```python
from build123d import *

# Parameters (mm, degrees)
EXTRUDE_1_DEPTH           = 50
FILLET_3_R                = 3
FILLET_4_R                = 3
EXTRUDE_4_DEPTH           = 60
EXTRUDE_5_DEPTH           = 62
CUT_EXTRUDE_7_DEPTH       = 63.635852353
CUT_EXTRUDE_7_DEPTH_BACK  = 4
SKETCH_8_R                = 3
EXTRUDE_6_DEPTH           = 25
CUT_EXTRUDE_10_DEPTH      = 67.695202226
CUT_EXTRUDE_10_DEPTH_BACK = 10


with BuildPart() as part:
    # 草图2 → 凸台-拉伸1 (new body)
    with BuildSketch(Plane(origin=(0, 0, 0), x_dir=(1, 0, 0), z_dir=(0, 1, 0))):
        with BuildLine():
            Line((25, -7.5), (22, -7.5))
            Line((22, -7.5), (22, -12.5))
            Line((22, -12.5), (30, -12.5))
            Line((30, -12.5), (30, 7.407682229))
            ThreePointArc((30, 7.407682229), (26.399187572, 8.899187572), (24.907682229, 12.5))
            Line((24.907682229, 12.5), (-25, 12.5))
            ThreePointArc((-25, 12.5), (-26.464466094, 8.964466094), (-30, 7.5))
            Line((-30, 7.5), (-30, -12.5))
            Line((-30, -12.5), (-22, -12.5))
            Line((-22, -12.5), (-22, -7.5))
            Line((-22, -7.5), (-25, -7.5))
            Line((-25, -7.5), (-25, 2.5))
            Line((-25, 2.5), (25, 2.5))
            Line((25, 2.5), (25, -7.5))
        make_face()
    extrude(amount=EXTRUDE_1_DEPTH)

    # 圆角3
    fillet_3_edges = [part.edges().sort_by_distance(p)[0] for p in [
        (-30, 25, -7.5),
        (-25, 25, -12.5),
    ]]
    fillet(fillet_3_edges, radius=FILLET_3_R)

    # 圆角4
    fillet_4_edges = [part.edges().sort_by_distance(p)[0] for p in [
        (24.907682229, 25, -12.5),
        (30, 25, -7.407682229),
    ]]
    fillet(fillet_4_edges, radius=FILLET_4_R)

    # 草图5 → 凸台-拉伸4 (add)
    with BuildSketch(Plane.ZY.offset(30)):
        Polygon((-2.5, 50), (-20.5, 50), (-2.5, 35), align=None)
    extrude(amount=-EXTRUDE_4_DEPTH)

    # 草图7 → 凸台-拉伸5 (add)
    with BuildSketch(Plane.ZY.offset(31)):
        with BuildLine():
            Line((-2.5, 51), (-2.5, 51.591557712))
            Line((-2.5, 51.591557712), (-2.5, 55))
            Line((-2.5, 55), (-3.5, 55))
            Line((-3.5, 55), (-3.5, 52))
            ThreePointArc((-3.5, 52), (-2.792893219, 51.707106781), (-2.5, 51))
        make_face()
        with BuildLine():
            ThreePointArc((-3.5, 50), (-2.792893219, 50.292893219), (-2.5, 51))
            ThreePointArc((-2.5, 51), (-2.792893219, 51.707106781), (-3.5, 52))
            Line((-3.5, 52), (-3.5, 51))
            Line((-3.5, 51), (-4.5, 51))
            ThreePointArc((-4.5, 51), (-4.207106781, 50.292893219), (-3.5, 50))
        make_face()
        with BuildLine():
            Line((-21.5, 50), (-3.5, 50))
            ThreePointArc((-3.5, 50), (-4.207106781, 50.292893219), (-4.5, 51))
            Line((-4.5, 51), (-21.5, 51))
            Line((-21.5, 51), (-21.5, 50))
        make_face()
    extrude(amount=-EXTRUDE_5_DEPTH)

    # 草图8 → 切除-拉伸7 (cut, two sides: drawn at the far end of the back side and taken through both)
    with BuildSketch(Plane(origin=(0, 50, 0), x_dir=(1, 0, 0), z_dir=(0, 1, 0)).offset(-CUT_EXTRUDE_7_DEPTH_BACK)):
        with Locations(Location((-15, 12.5, 0), (0, 0, 90))):
            Circle(SKETCH_8_R)
        with Locations(Location((15, 12.5, 0), (0, 0, 90))):
            Circle(SKETCH_8_R)
    extrude(amount=CUT_EXTRUDE_7_DEPTH + CUT_EXTRUDE_7_DEPTH_BACK, mode=Mode.SUBTRACT)

    # 草图9 → 凸台-拉伸6 (add)
    with BuildSketch(Plane(origin=(0, 0, 0), x_dir=(1, 0, 0), z_dir=(0, 1, 0))):
        with BuildLine():
            Line((-5, -17.5), (5, -17.5))
            ThreePointArc((5, -17.5), (8.535533906, -16.035533906), (10, -12.5))
            Line((10, -12.5), (10, 2.5))
            Line((10, 2.5), (-10, 2.5))
            Line((-10, 2.5), (-10, -12.5))
            ThreePointArc((-10, -12.5), (-8.535533906, -16.035533906), (-5, -17.5))
        make_face()
    extrude(amount=EXTRUDE_6_DEPTH)

    # 草图9<8> → 切除-拉伸10 (cut, two sides: drawn at the far end of the back side and taken through both)
    with BuildSketch(Plane(origin=(0, 0, 0), x_dir=(1, 0, 0), z_dir=(0, 1, 0)).offset(-CUT_EXTRUDE_10_DEPTH_BACK)):
        with BuildLine():
            ThreePointArc((0, -1.5), (-6, -7.5), (0, -13.5))
            Line((0, -13.5), (0, -7.5))
            Line((0, -7.5), (0, -1.5))
        make_face()
        with BuildLine():
            Line((0, -7.5), (0, -13.5))
            ThreePointArc((0, -13.5), (4.242640687, -11.742640687), (6, -7.5))
            ThreePointArc((6, -7.5), (4.242640687, -3.257359313), (0, -1.5))
            Line((0, -1.5), (0, -7.5))
        make_face()
    extrude(amount=CUT_EXTRUDE_10_DEPTH + CUT_EXTRUDE_10_DEPTH_BACK, mode=Mode.SUBTRACT)


solid = part.part
```
Source: CAD feature listing. Evaluate the final solid. Frame: model axes, mm. A direction names the side the tool comes from. Round coordinates to 2 decimals unless told otherwise and drop trailing zeros. Loops run counter-clockwise (first coordinate to the right, second up) from the corner with the lowest first, then second, coordinate; pieces in that order, holes last.
1. Section query A-A on x = 24. Output: boundary loops of the cut face in (y, z).
2. Contact query for flat-ended pins moving along their axis: pin 1 (3 mm diameter, centred on x = -2.5, z = -11, fed in from +Y); pin 2 (3 mm diameter, centred on x = 4, y = 33.5, fed in from +Z); pin 3 (2.5 mm diameter, centred on x = 24.5, y = 28, fed in from +Z); pin 4 (3 mm diameter, centred on x = 15.5, z = -0.5, fed in from -Y). Output: stop coordinate, or through.
3. Ray query, L1, parallel to X at y = 48.25, z = -12.5; L2, parallel to X at y = 30.5, z = 2; L3, parallel to X at y = 5.5, z = 5. Return the intervals inside material, ascending.
4. Section query B-B on z = 11. Output: boundary loops of the cut face in (x, y), and give its area (3 significant figures).
5. Mould query, pull axis X, two halves, no side actions, for faces 5 (the flat face through (0, 30, -2.5)), 6 (the cylindrical face through (8.5, 12.32, 16.07)), 7 (the flat face through (-0.4, 46.5, -16.3)). Classes: released by +X, released by -X, zero draft, split by the parting line, or undercut.
6. Section query C-C on y = 33. Output: boundary loops of the cut face in (x, z) (3 decimals).
7. Section query D-D on x = 15. Output: boundary loops of the cut face in (y, z).
8. Access query for faces 1 (the flat face through (0, 53, -3.5)), 2 (the flat face through (0, 53, -2.5)), 3 (the cylindrical face through (17.93, 48.46, -11.85)), 4 (the cylindrical face through (29.47, 19.97, -6.69)). Directions: +Z, -Z, +X, -X, +Y, -Y. A direction counts if a zero-diameter tool reaches every point of the face in a straight line with its end or side. Return the directions, or none.
Answers below:
1. outline: (0, -12.09) - (42.99, -12.09) - (50, -20.5) - (50, -21.5) - (51, -21.5) - (51, -3.5) - (55, -3.5) - (55, -2.5) - (51, -2.5) arc R1 ccw to (50, -3.5) - (50, -2.5) - (0, -2.5) - close; (0, 7.5) - (50, 7.5) - (50, 12.5) - (0, 12.5) - close
2. pin 1: stops at y = 51
2. pin 2: stops at z = -2.5
2. pin 3: stops at z = 12.5
2. pin 4: passes through
3. L1: x = -30 to -18, -12 to 12, 18 to 30
3. L2: x = -30 to -25, 25 to 30
3. L3: x = -30 to -25, -10 to -5.45, 5.45 to 10, 25 to 30
4. outline: (-30, 0) - (-22, 0) - (-22, 50) - (-30, 50) - close; (-10, 0) - (-4.87, 0) - (-4.87, 25) - (-10, 25) - close; (4.87, 0) - (10, 0) - (10, 25) - (4.87, 25) - close; (22, 0) - (30, 0) - (30, 50) - (22, 50) - close
4. area: 1,060 mm2
5. face 5: undercut
5. face 6: released by +X
5. face 7: zero draft
6. outline: (-30, -5.084) arc R3 ccw to (-28.125, -7.865) arc R5 cw to (-25.365, -10.625) arc R3 ccw to (-22.584, -12.5) - (22.484, -12.5) arc R3 ccw to (25.271, -10.612) arc R5.092 cw to (28.112, -7.771) arc R3 ccw to (30, -4.984) - (30, 12.5) - (22, 12.5) - (22, 7.5) - (25, 7.5) - (25, -2.5) - (-25, -2.5) - (-25, 7.5) - (-22, 7.5) - (-22, 12.5) - (-30, 12.5) - close
7. outline: (0, -12.5) - (43.33, -12.5) - (50, -20.5) - (50, -21.5) - (51, -21.5) - (51, -15.5) - (46, -15.5) - (46, -9.5) - (51, -9.5) - (51, -3.5) - (55, -3.5) - (55, -2.5) - (51, -2.5) arc R1 ccw to (50, -3.5) - (50, -2.5) - (0, -2.5) - close
8. face 1: -Z, +X, -X, +Y
8. face 2: +Z, +X, -X, +Y
8. face 3: +Y
8. face 4: -Z, +X, -Y
